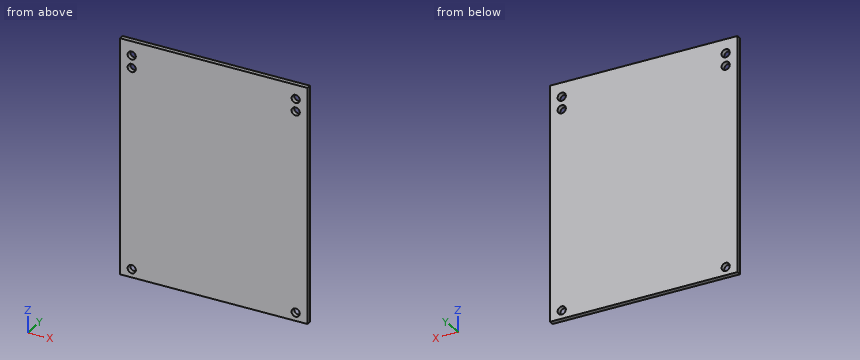
Autodesk Fusion 360 part; units mm, degrees
sketch "スケッチ1" plane through (0, 0, 0) normal (0, 1, 0) x (1, 0, 0)
  line L0 (-40, -50) -> (40, -50)
  line L1 (40, -50) -> (40, 50)
  line L2 (40, 50) -> (-40, 50)
  line L3 (-40, 50) -> (-40, -50)
  line L4 (-40, -50) -> (40, 50) construction
  line L5 (40, -50) -> (-40, 50) construction
  dimension "d1" = 80
  dimension "d2" = 100
extrude "押し出し1" add sketch "スケッチ1" along normal blind 2
sketch "スケッチ2" plane through (0, 2, 0) normal (0, 1, 0) x (-1, 0, 0)
  line L0 (40, -50) -> (40, 50)
  line L1 (40, 50) -> (-40, 50)
  line L2 (-40, 50) -> (-40, -50)
  line L3 (-40, -50) -> (40, -50)
  line L4 (0, -50) -> (0, -46.5)
  line L5 (0, -46.5) -> (35, -46.5)
  line L6 (0, -46.5) -> (-35, -46.5)
  circle A0 centre (35, -46.5) radius 1.75
  circle A1 centre (-35, -46.5) radius 1.75
  line L7 (35, -46.5) -> (35, 44)
  circle A2 centre (35, 44) radius 1.75
  line L8 (35, 44) -> (-35, 44)
  circle A3 centre (-35, 44) radius 1.75
  dimension "d5" = 3.5
  dimension "d6" = 35
  dimension "d7" = 35
  dimension "d8" = 3.5
  dimension "d9" = 3.5
  dimension "d10" = 90.5
  dimension "d11" = 3.5
  dimension "d12" = 70
  dimension "d13" = 3.5
extrude "押し出し2" cut sketch "スケッチ2" against normal blind 5 contours A1 | A3 | L7 A2 L8 | L7 A2 L8 | L5 A0 L7 | L5 A0 L7
sketch "スケッチ3" plane through (0, 2, 0) normal (0, 1, 0) x (-1, 0, 0)
  circle A0 centre (35, -46.5) radius 1.75
  circle A1 centre (35, 44) radius 1.75
  circle A2 centre (-35, -46.5) radius 1.75
  circle A3 centre (-35, 44) radius 1.75
  line L0 (40, -50) -> (40, 50)
  line L1 (40, 50) -> (-40, 50)
  line L2 (-40, 50) -> (-40, -50)
  line L3 (-40, -50) -> (40, -50)
  line L4 (35, 44) -> (35, 38.71)
  line L5 (-35, 44) -> (-35, 38.71)
  circle A4 centre (35, 38.71) radius 1.75
  circle A5 centre (-35, 38.71) radius 1.75
  dimension "d16" = 5.29
  dimension "d17" = 5.29
  dimension "d18" = 3.5
  dimension "d19" = 3.5
extrude "押し出し3" cut sketch "スケッチ3" against normal blind 14 contours A4 | A5
Source: CAD feature listing. Evaluate the final solid. Frame: model axes, mm. Give positions to 0.01 mm unless a question says otherwise; leave off trailing zeros. Write each loop counter-clockwise with the first axis right and the second up, starting at its lowest first coordinate (ties: lowest second). Pieces come first, ordered by that corner, then holes. Notation, with made-up numbers: M -30,53 L 25,53 A20 cw 25,69 Z; hole C 37,56.25 d2. An arc over 180 degrees is marked long. Answer as a JSON object with one key per item and string values.
Q1. Contact query for a flat-ended pin moving along its axis: P1, Ø3, axis at x = -35, z = 44, coming from the -Y side. Output: stop coordinate, or through.
Geometry check:
{"P1": "passes through"}
Q2. Cut plane A-A, the plane x = -35. Return the cut outline in (y, z).
Geometry check:
{"outline": "M 0,-50 L 2,-50 L 2,-48.25 L 0,-48.25 Z; M 0,-44.75 L 2,-44.75 L 2,36.96 L 0,36.96 Z; M 0,40.46 L 2,40.46 L 2,42.25 L 0,42.25 Z; M 0,45.75 L 2,45.75 L 2,50 L 0,50 Z"}
Q3. Ray query, line 1 along Z through (x, y) = (35, 1.05); line 2 along X through (y, z) = (0.6, 38.71); line 3 along X through (y, z) = (0.85, 38). Return the intervals inside material, ascending.
Geometry check:
{"line 1": "z = -50 to -48.25, -44.75 to 36.96, 40.46 to 42.25, 45.75 to 50", "line 2": "x = -40 to -36.75, -33.25 to 33.25, 36.75 to 40", "line 3": "x = -40 to -36.6, -33.4 to 33.4, 36.6 to 40"}
Q4. Cut plane B-B, the plane z = 38.71. Return the cut outline in (x, y), then the cut area to 3 significant figures.
Geometry check:
{"outline": "M -40,0 L -36.75,0 L -36.75,2 L -40,2 Z; M -33.25,0 L 33.25,0 L 33.25,2 L -33.25,2 Z; M 36.75,0 L 40,0 L 40,2 L 36.75,2 Z", "area": "146 mm^2"}
